```python
from build123d import *

# Parameters (mm, degrees)
EXTRUDE_1_DEPTH     = 6.3
SKETCH_2_R          = 6.3
SKETCH_2_R_2        = 2.9
EXTRUDE_2_DEPTH     = 2.2
EXTRUDE_START       = 2.2
SKETCH_2_3_R        = 2.9
EXTRUDE_3_DEPTH     = 5.8
SKETCH_3_R          = 1.5
CUT_EXTRUDE_1_DEPTH = 5.8


with BuildPart() as part:
    # Эскиз1 → Бобышка-Вытянуть1 (new, symmetric)
    with BuildSketch(Plane.XY):
        Polygon((-11.65, -11.85), (11.65, -11.85), (11.65, 3.15), (14.95, 3.15), (14.95, 5.15), (11.65, 5.15), (11.65, 11.85), (-11.65, 11.85), (-11.65, 5.15), (-14.95, 5.15), (-14.95, 3.15), (-11.65, 3.15), align=None)
    extrude(amount=EXTRUDE_1_DEPTH, both=True)

    # Эскиз2 → Бобышка-Вытянуть2 (add)
    with BuildSketch(Plane(origin=(0, 11.85, 0), x_dir=(1, 0, 0), z_dir=(0, 1, 0))):
        with Locations(Location((5.35, 0, 0), (0, 0, 270))):
            Circle(SKETCH_2_R)
        with Locations((5.35, 0)):
            Circle(SKETCH_2_R_2, mode=Mode.SUBTRACT)
        with Locations((5.35, 0)):
            Circle(SKETCH_2_R_2)
    extrude(amount=EXTRUDE_2_DEPTH)

    # Эскиз2<3> → Бобышка-Вытянуть3 (add)
    with BuildSketch(Plane(origin=(0, 11.85, 0), x_dir=(1, 0, 0), z_dir=(0, 1, 0)).offset(EXTRUDE_START)):
        with Locations(Location((5.35, 0, 0), (0, 0, 180))):
            Circle(SKETCH_2_3_R)
    extrude(amount=EXTRUDE_3_DEPTH)

    # Эскиз3 → Вырез-Вытянуть1 (cut)
    with BuildSketch(Plane(origin=(0, 5.15, 0), x_dir=(1, 0, 0), z_dir=(0, 1, 0))):
        with Locations(Location((-13.3, 0, 0), (0, 0, 270))):
            Circle(SKETCH_3_R)
        with Locations(Location((13.3, 0, 0), (0, 0, 180))):
            Circle(SKETCH_3_R)
    extrude(amount=-CUT_EXTRUDE_1_DEPTH, mode=Mode.SUBTRACT)


solid = part.part
```
Check sheet for the modelled part. Datum: model origin and axes. Units: mm. A direction names the side the tool comes from. Give positions to 0.01 mm unless a question says otherwise; leave off trailing zeros. Write each loop counter-clockwise with the first axis right and the second up, starting at its lowest first coordinate (ties: lowest second). Pieces come first, ordered by that corner, then holes. Notation, with made-up numbers: (12.25, 73.5) -> (22.25, 73.5) arc R15 cw to (22.25, 83.5) -> close; hole circle Ø7 at (10, -27.75). An arc over 180 degrees is marked (long way). Use CSV: the item, a comma, the result in double quotes. Start each with the question number.
Q1. Tool access check on faces 1 (the flat face through (11.65, 8, 0)), 2 (the flat face through (-14.1, 3.15, 1.5)), 3 (the cylindrical face through (-0.239, 12.935, 2.907)), 4 (the flat face through (-11.65, 9, 0)). Record the directions out of +Z, -Z, +X, -X, +Y, -Y that give a thin tool (end or side, any length) a straight path to the whole face; none if there is none.
Q2. Cross-section at A-A on x = -13.3. Enter the section's corners in (y, z), and give its area (3 significant figures).
Q3. Scan lines: line 1 along Y through (x, z) = (-4, -1.5); line 2 along Z through (x, y) = (13.3, 4); line 3 along Y through (x, z) = (9.25, 0.75). Record each from-to range of solid material in increasing order.
Q4. Cross-section at C-C on y = -4.5. Enter the section's corners in (x, z).
Q5. Depth check by flat-ended pin: P1, Ø3.5, axis at x = -13.5, z = 3, coming from the -Y side; P2, Ø1, axis at x = -13.5, z = -1.5, coming from the +Y side; P3, Ø2, axis at y = 9.5, z = 1, coming from the +X side; P4, Ø1, axis at x = 12.5, z = -0.5, coming from the -Y side. Enter the tip coordinate at first touch or a pass-through.
Q6. Cross-section at B-B on x = 0.25. Enter the section's corners in (y, z).
Working result:
1,face 1,"+Z, -Z, +X, +Y"
1,face 2,"+Z, -Z, -X, -Y"
1,face 3,"+Y"
1,face 4,"+Z, -Z, -X, +Y"
2,outline,"(3.15, -6.3) -> (5.15, -6.3) -> (5.15, -1.5) -> (3.15, -1.5) -> close; (3.15, 1.5) -> (5.15, 1.5) -> (5.15, 6.3) -> (3.15, 6.3) -> close"
2,area,"19.2 mm^2"
3,line 1,"y = -11.85 to 11.85"
3,line 2,"z = -6.3 to -1.5, 1.5 to 6.3"
3,line 3,"y = -11.85 to 14.05"
4,outline,"(-11.65, -6.3) -> (11.65, -6.3) -> (11.65, 6.3) -> (-11.65, 6.3) -> close"
5,P1,"stops at y = 3.15"
5,P2,"stops at y = 5.15"
5,P3,"stops at x = 11.65"
5,P4,"passes through"
6,outline,"(-11.85, -6.3) -> (11.85, -6.3) -> (11.85, -3.7) -> (14.05, -3.7) -> (14.05, 3.7) -> (11.85, 3.7) -> (11.85, 6.3) -> (-11.85, 6.3) -> close"
